CAD build for the part. Positions are in the model's coordinates, mm. A direction names the side the tool comes from. Round coordinates to 2 decimals unless told otherwise and drop trailing zeros. Loops run counter-clockwise (first coordinate to the right, second up) from the corner with the lowest first, then second, coordinate; pieces in that order, holes last. Notation, with made-up numbers: M 73.25,-18 L 109.25,-18 A18 cw 109.25,-5 Z; hole C -33,-2 d10. An arc over 180 degrees is marked long. Use one line per item in the form item = value.
from build123d import *

# Parameters (mm, degrees)
BOSS_EXTRUDE1_DEPTH = 10


with BuildPart() as part:
    # Sketch1 → Boss-Extrude1 (new body)
    with BuildSketch(Plane.XY):
        with BuildLine():
            Line((125, 175), (50, 175))
            ThreePointArc((50, 175), (43.301270189, 150), (25, 131.698729811))
            Line((25, 131.698729811), (25, -68.301270189))
            ThreePointArc((25, -68.301270189), (0, -93.301270189), (-25, -68.301270189))
            Line((-25, -68.301270189), (-25, 131.698729811))
            ThreePointArc((-25, 131.698729811), (-43.301270189, 150), (-50, 175))
            Line((-50, 175), (-125, 175))
            Line((-125, 175), (-175, 125))
            Line((-175, 125), (-175, -125))
            Line((-175, -125), (-125, -175))
            Line((-125, -175), (-50, -175))
            ThreePointArc((-50, -175), (0, -125), (50, -175))
            Line((50, -175), (125, -175))
            Line((125, -175), (175, -125))
            Line((175, -125), (175, 125))
            Line((175, 125), (125, 175))
        make_face()
    extrude(amount=BOSS_EXTRUDE1_DEPTH)


solid = part.part
1. Tool access for faces 4 (the face through (43.483, 150.318, 4.93)), 5 (the face through (-41, 2, 10)): list every direction of +Z, -Z, +X, -X, +Y, -Y with a clear straight run to the whole face (end or side of a thin tool).
Completed:
face_4 = +Z, -Z, +Y
face_5 = +Z, +X, -X, +Y, -Y
2. Drop flat-ended pins along their axis: P1, Ø3, axis at x = 37.5, z = 3.5, coming from the +Y side; P2, Ø8, axis at x = 17.5, y = -32.5, coming from the -Z side. Give the stop position or say it passes through.
Completed:
P1 = 143.71
P2 = through
3. Cut at D-D on x = -137. Write the cut outline in (y, z).
Completed:
outline = M -163,0 L 163,0 L 163,10 L -163,10 Z
4. Pull direction X, two halves, no side cores. Call faces 1 (the face through (88, 175, 5)), 2 (the face through (150, -150, 5)), 3 (the face through (25, 33, 5)): +X half, -X half, draft (parallel to the pull), parting line (faces both ways), or undercut.
Completed:
face_1 = draft
face_2 = +X half
face_3 = undercut
5. Probe line 1 along X through (y, z) = (93.5, 0.5); line 2 along X through (y, z) = (138, 5.25); line 3 along Y through (x, z) = (33, 8). List the from-to ranges inside material, lowest first. Write a range as from..to.
Completed:
line_1 = -175..-25, 25..175
line_2 = -162..-33.63, 33.63..162
line_3 = -137.44..137.44
6. Cut at A-A on y = -22.5. Write the cut outline in (x, z), and give its area (3 significant figures).
Completed:
outline = M -175,0 L -25,0 L -25,10 L -175,10 Z; M 25,0 L 175,0 L 175,10 L 25,10 Z
area = 3,000 mm2
7. Cut at B-B on z = 3. Write the cut outline in (x, y), and give its area (3 significant figures).
Completed:
outline = M -175,-125 L -125,-175 L -50,-175 A50 cw 50,-175 L 125,-175 L 175,-125 L 175,125 L 125,175 L 50,175 A50 cw 25,131.7 L 25,-68.3 A25 cw -25,-68.3 L -25,131.7 A50 cw -50,175 L -125,175 L -175,125 Z
area = 98,900 mm2
8. Cut at C-C on x = 143. Write the cut outline in (y, z).
Completed:
outline = M -157,0 L 157,0 L 157,10 L -157,10 Z
